Could you check a few things on this drawing? It's one solid part, dimensions in mm from its lowest x, y, z. Round coordinates to 2 decimals unless told otherwise and drop trailing zeros. Put each result on its own line as item: value.
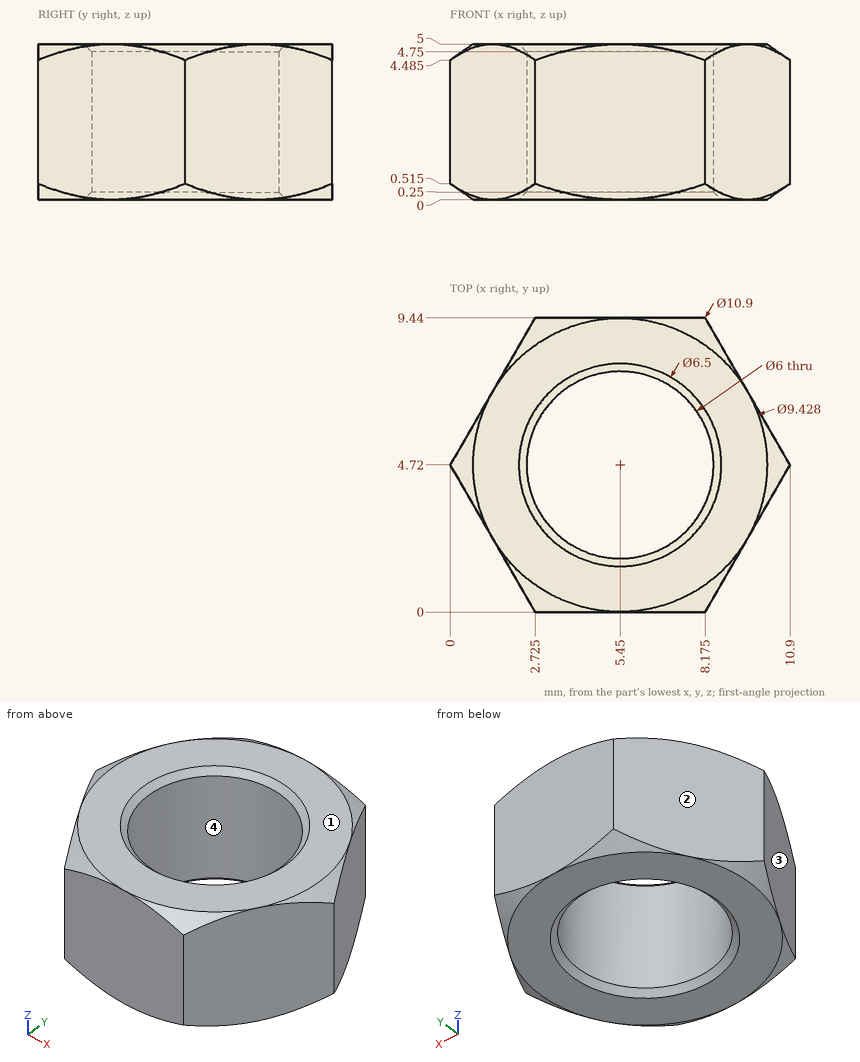
(1) Please list where these lines run through material, in increasing order: probe 1 along Y at (x, z) = (5.5, 4.25); probe 2 along X at (y, z) = (4, 1.7) (1 decimal); probe 3 along X at (y, z) = (3.75, 0.9). Write a range as from..to.
Values found:
probe 1: y = 0..1.72, 7.72..9.44
probe 2: x = 0.4..2.5, 8.4..10.5
probe 3: x = 0.56..2.61, 8.29..10.34
(2) If we mould it in two halves opening along Y, with no side actions, what happens to the marked faces 1, 2, 3 and 4? For each: pulls with the +Y half, pulls with the -Y half, needs draft (parallel to the pull), parting line crosses it, or undercut.
Values found:
face 1: needs draft
face 2: pulls with the +Y half
face 3: pulls with the -Y half
face 4: undercut
(3) I'm going to push flat-ended pins straight in: pin 1 (3 mm diameter, centred on y = 1.5, z = 1, fed in from -X); pin 2 (1 mm diameter, centred on y = 8.5, z = 2, fed in from +X); pin 3 (1 mm diameter, centred on y = 3, z = 2, fed in from -X) (1 decimal). Where does each tip first touch, or does it pass through?
Values found:
pin 1: stops at x = 0.99
pin 2: stops at x = 9.01
pin 3: stops at x = 0.7
